Design review of the part built by this model. Coordinates are the model's own, in mm. Coordinates: 2 decimals unless noted, no trailing zeros. Loops run counter-clockwise (first coordinate to the right, second up) from the corner with the lowest first, then second, coordinate; pieces in that order, holes last. Notation, with made-up numbers: M -23,6.25 L -19,6.25 A18 cw -19,25.25 Z; hole C 3,81.5 d1. An arc over 180 degrees is marked long. Put each result on its own line as item: value. Start each with the question number.
(1) Clearance check with a flat-ended pin moving along its axis: pin 1 (2 mm diameter, centred on x = 143.4, y = 253.8, fed in from -Z). State where the tip first meets the part, or that it passes through.
(2) Take a section at B-B, the plane z = 2.55. Give the boundary of the cut face in (x, y).
(3) Take a section at A-A, the plane x = 178. Give the boundary of the cut face in (y, z).
(4) For probe 1 along Y at (x, z) = (190, 0.2); probe 2 along X at (y, z) = (303.5, 1.3); probe 3 along X at (y, z) = (304.5, 1.35), list the stretches that pass through material, from the lowest coordinate up. Write a range as [from, to].
```python
from build123d import *

# Parameters (mm, degrees)
ESQUISSE1_R        = 1.345345221
ESQUISSE1_R_2      = 1.346909221
ESQUISSE1_R_3      = 1.298611316
ESQUISSE1_R_4      = 1.335683761
ESQUISSE1_W        = 51.06055426
ESQUISSE1_H        = 5.162843369
BOSS_EXTRU_1_DEPTH = 3


with BuildPart() as part:
    # Esquisse1 → Boss.-Extru.1 (new body)
    with BuildSketch(Plane.XY):
        with BuildLine():
            Line((142.914343154, 306.333520822), (201.871913252, 306.333520822))
            ThreePointArc((201.871913252, 306.333520822), (203.993233595, 305.454841166), (204.871913252, 303.333520822))
            Line((204.871913252, 303.333520822), (204.871913252, 253.348131253))
            ThreePointArc((204.871913252, 253.348131253), (203.993233595, 251.22681091), (201.871913252, 250.348131253))
            Line((201.871913252, 250.348131253), (142.914343154, 250.348131253))
            ThreePointArc((142.914343154, 250.348131253), (140.793022811, 251.22681091), (139.914343154, 253.348131253))
            Line((139.914343154, 253.348131253), (139.914343154, 303.333520822))
            ThreePointArc((139.914343154, 303.333520822), (140.793022811, 305.454841166), (142.914343154, 306.333520822))
        make_face()
        with Locations((143.360544481, 302.831604494)):
            Circle(ESQUISSE1_R, mode=Mode.SUBTRACT)
        with Locations((201.344684378, 302.818633302)):
            Circle(ESQUISSE1_R_2, mode=Mode.SUBTRACT)
        with Locations((143.395469299, 253.802031827)):
            Circle(ESQUISSE1_R_3, mode=Mode.SUBTRACT)
        with Locations((201.354862046, 253.815125268)):
            Circle(ESQUISSE1_R_4, mode=Mode.SUBTRACT)
        with Locations((172.371550879, 302.856687584)):
            Rectangle(ESQUISSE1_W, ESQUISSE1_H, mode=Mode.SUBTRACT)
    extrude(amount=BOSS_EXTRU_1_DEPTH)


solid = part.part
```
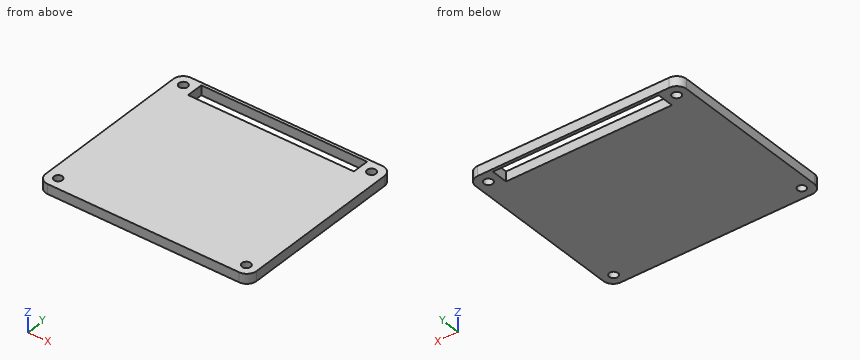
Computed values:
1. pin 1: passes through
2. outline: M 139.91,253.35 A3 ccw 142.91,250.35 L 201.87,250.35 A3 ccw 204.87,253.35 L 204.87,303.33 A3 ccw 201.87,306.33 L 142.91,306.33 A3 ccw 139.91,303.33 Z; hole C 143.36,302.83 d2.69; hole C 143.4,253.8 d2.6; hole M 146.84,300.28 L 197.9,300.28 L 197.9,305.44 L 146.84,305.44 Z; hole C 201.34,302.82 d2.69; hole C 201.35,253.82 d2.67
3. outline: M 250.35,0 L 300.28,0 L 300.28,3 L 250.35,3 Z; M 305.44,0 L 306.33,0 L 306.33,3 L 305.44,3 Z
4. probe 1: y = [250.35, 300.28], [305.44, 306.33]
4. probe 2: x = [139.92, 142.19], [144.53, 146.84], [197.9, 200.18], [202.51, 204.87]
4. probe 3: x = [140.15, 146.84], [197.9, 204.64]
